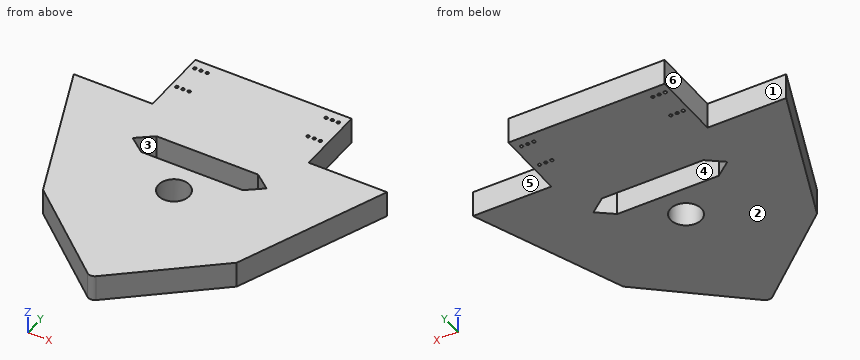
from build123d import *

# Parameters (mm, degrees)
F0_R     = 15
F0_R_2   = 1.5
F1_DEPTH = 25.4


with BuildPart() as f1:
    # F0 (on Top) → F1 (new body)
    with BuildSketch(Plane.XY):
        with BuildLine():
            Line((77.3958978424, 102.9117530549), (-74.8905959537, 102.9117530549))
            Line((-74.8905959537, 102.9117530549), (-74.8905959537, 33.9117530549))
            Line((-74.8905959537, 33.9117530549), (-93.1560286085, 25.7647309037))
            Line((-93.1560286085, 25.7647309037), (-93.1560286085, -111.9823026415))
            Line((-93.1560286085, -111.9823026415), (-3.4501732079, -188.27225021))
            ThreePointArc((-3.4501732079, -188.27225021), (0.6432284934, -189.7849664775), (4.7462730705, -188.2986040749))
            Line((4.7462730705, -188.2986040749), (95.6613304972, -111.9823026415))
            Line((95.6613304972, -111.9823026415), (95.6613304972, 25.7647309037))
            Line((95.6613304972, 25.7647309037), (77.3958978424, 33.9117530549))
            Line((77.3958978424, 33.9117530549), (77.3958978424, 102.9117530549))
        make_face()
        with Locations((0.6369164785, -56.0882469451)):
            Circle(F0_R, mode=Mode.SUBTRACT)
        Polygon((-49.4758075681, -26.1185521963), (-65.2628552972, -13.8397442737), (-49.4758075681, -1.5609363511), (49.5241924319, -1.5609363511), (65.311240161, -13.8397442737), (49.5241924319, -26.1185521963), align=None, mode=Mode.SUBTRACT)
        with Locations((-69.3630835215, 63.9117530549)):
            Circle(F0_R_2, mode=Mode.SUBTRACT)
        with Locations((-63.3630835215, 63.9117530549)):
            Circle(F0_R_2, mode=Mode.SUBTRACT)
        with Locations((-57.3630835215, 63.9117530549)):
            Circle(F0_R_2, mode=Mode.SUBTRACT)
        with Locations((-69.3630835215, 92.9117530549)):
            Circle(F0_R_2, mode=Mode.SUBTRACT)
        with Locations((-63.3630835215, 92.9117530549)):
            Circle(F0_R_2, mode=Mode.SUBTRACT)
        with Locations((-57.3630835215, 92.9117530549)):
            Circle(F0_R_2, mode=Mode.SUBTRACT)
        with Locations((58.6369164785, 63.9117530549)):
            Circle(F0_R_2, mode=Mode.SUBTRACT)
        with Locations((64.6369164785, 63.9117530549)):
            Circle(F0_R_2, mode=Mode.SUBTRACT)
        with Locations((70.6369164785, 63.9117530549)):
            Circle(F0_R_2, mode=Mode.SUBTRACT)
        with Locations((58.6369164785, 92.9117530549)):
            Circle(F0_R_2, mode=Mode.SUBTRACT)
        with Locations((64.6369164785, 92.9117530549)):
            Circle(F0_R_2, mode=Mode.SUBTRACT)
        with Locations((70.6369164785, 92.9117530549)):
            Circle(F0_R_2, mode=Mode.SUBTRACT)
        Polygon((-93.1560286085, 25.7647309037), (-74.8905959537, 33.9117530549), (-151.5982151031, 33.9117530549), (-93.1560286085, -111.9823026415), align=None)
        Polygon((153.7487208843, 33.9117530549), (77.3958978424, 33.9117530549), (95.6613304972, 25.7647309037), (95.6613304972, -111.9823026415), align=None)
    extrude(amount=F1_DEPTH)


solid = f1.part
The listing builds one solid part. Answer for the finished solid, in the listing's coordinates (mm). Face numbers are marked on the shaded views. A direction names the side the tool comes from. Give positions to 0.01 mm unless a question says otherwise; leave off trailing zeros. Loops run counter-clockwise (first coordinate to the right, second up) from the corner with the lowest first, then second, coordinate; pieces in that order, holes last. Notation, with made-up numbers: (78.25, 14.5) - (86.25, 14.5) arc R20 cw to (86.25, 33.5) - close; hole circle Ø6 at (-31, -36). An arc over 180 degrees is marked (long way). Answer as a JSON object with one key per item and string values.
1. A cutting plane is placed at C-C (z = 6). Give the number of separate pieces and of enclosed holes in the cut face, then the cut area to 3 significant figures.
Determined:
{"separate pieces": "1", "enclosed holes": "14", "area": "50,500 mm²"}
2. Flat-ended cylindrical pins translate along their axes: pin 1 Ø8 at (x, z) = (87, 10.5) entering from +Y; pin 2 Ø1 at (x, z) = (-28.5, 14) entering from -Y; pin 3 Ø4 at (y, z) = (-53, 7.5) entering from -X. Find the tip coordinate at first contact, or state that the pin passes through.
Determined:
{"pin 1": "y = 33.91", "pin 2": "y = -167.39", "pin 3": "x = -117.58"}
3. A cutting plane is placed at A-A (y = -65). Write down the section's boundary in (x, z), then the cut area to 3 significant figures.
Determined:
{"outline": "(-111.98, 0) - (-11.43, 0) - (-11.43, 25.4) - (-111.98, 25.4) - close; (12.7, 0) - (114.37, 0) - (114.37, 25.4) - (12.7, 25.4) - close", "area": "5,140 mm²"}
4. For the marked faces 4, 5 and 6, determine the directions among +Z, -Z, +X, -X, +Y, -Y from which every point of the face is accessible in a straight line to the end or side of a thin tool.
Determined:
{"face 4": "+Z, -Z", "face 5": "+Z, -Z, +X, +Y", "face 6": "+Z, -Z, -X, +Y"}
5. A cutting plane is placed at D-D (y = 58.5). Write down the section's boundary in (x, z), then the cut area to 3 significant figures.
Determined:
{"outline": "(-74.89, 0) - (77.4, 0) - (77.4, 25.4) - (-74.89, 25.4) - close", "area": "3,870 mm²"}
6. Find the intervals of material crossed by L1, parallel to Y at x = 12, z = 5.5; L2, parallel to Y at x = 1, z = 14.25; L3, parallel to Y at x = -43.5, z = 11, in increasing order. Write a range as [from, to].
Determined:
{"L1": "[-182.21, -65.88], [-46.3, -26.12], [-1.56, 102.91]", "L2": "[-189.78, -71.08], [-41.09, -26.12], [-1.56, 102.91]", "L3": "[-154.21, -26.12], [-1.56, 102.91]"}
7. For a pull along Y with two mould halves and no side action, classify the marked faces 1, 2 and 3 as pulls with the +Y half, pulls with the -Y half, needs draft (parallel to the pull), parting line crosses it, or undercut.
Determined:
{"face 1": "pulls with the +Y half", "face 2": "needs draft", "face 3": "undercut"}
8. A cutting plane is placed at B-B (x = 0). Write down the section's boundary in (y, z), then the cut area to 3 significant figures.
Determined:
{"outline": "(-189.75, 0) - (-71.07, 0) - (-71.07, 25.4) - (-189.75, 25.4) - close; (-41.1, 0) - (-26.12, 0) - (-26.12, 25.4) - (-41.1, 25.4) - close; (-1.56, 0) - (102.91, 0) - (102.91, 25.4) - (-1.56, 25.4) - close", "area": "6,050 mm²"}
